from build123d import *

# Parameters (mm, degrees)
F_10_0MM_DOWEL_HOLE1_D      = 15
F_10_0MM_DOWEL_HOLE1_DEPTH  = 12
CIRPATTERN1_COUNT           = 6
F_10_0MM_DOWEL_HOLE2_D      = 15
F_10_0MM_DOWEL_HOLE2_DEPTH  = 12
CIRPATTERN2_COUNT           = 6
BOSS_EXTRUDE1_REACH         = 220.918
BOSS_EXTRUDE1_END_RADIUS    = 75
SKETCH12_R                  = 45
F_10_0MM_DOWEL_HOLE3_REACH  = 287.526
F_10_0MM_DOWEL_HOLE3_BORE_R = 30
F_12_0MM_DOWEL_HOLE1_D      = 12
F_12_0MM_DOWEL_HOLE1_DEPTH  = 12
CIRPATTERN3_COUNT           = 6


with BuildPart() as part:
    # Sketch1 → Revolve1 (revolve)
    with BuildSketch(Plane.XY, mode=Mode.PRIVATE) as revolve1_sk:
        Polygon((-100, -52.5), (-100, -95), (-88, -95), (-88, -62.5), (-50, -62.5), (-50, -75), (50, -75), (50, -65), (74, -65), (74, -50), (88, -50), (88, -95), (100, -95), (100, -36), (54, -36), (54, -43.5), (37, -43.5), (37, -52.5), (-35, -52.5), (-35, -47.5), (-95, -47.5), (-95, -52.5), align=None)
    revolve(revolve1_sk.sketch.rotate(Axis((0, 0, 0), (1, 0, 0)), 270), axis=Axis((0, 0, 0), (1, 0, 0)))

    # Ø10.0mm Dowel Hole1
    with Locations(Plane(origin=(100, 0, 0), x_dir=(0, 0, -1), z_dir=(1, 0, 0))):
        with Locations((0, 75)):
            f_10_0mm_dowel_hole1 = Hole(F_10_0MM_DOWEL_HOLE1_D / 2, depth=F_10_0MM_DOWEL_HOLE1_DEPTH)

    # CirPattern1: Ø10.0mm Dowel Hole1 ×6 about axis
    cirpattern1_axis = Axis((0, 0, 0), (1, 0, 0))
    for i in range(1, CIRPATTERN1_COUNT):
        add(f_10_0mm_dowel_hole1.rotate(cirpattern1_axis, i * 360 / CIRPATTERN1_COUNT), mode=Mode.SUBTRACT)

    # Ø10.0mm Dowel Hole2
    with Locations(Plane.ZY.offset(100)):
        with Locations((75, 0)):
            f_10_0mm_dowel_hole2 = Hole(F_10_0MM_DOWEL_HOLE2_D / 2, depth=F_10_0MM_DOWEL_HOLE2_DEPTH)

    # CirPattern2: Ø10.0mm Dowel Hole2 ×6 about axis
    cirpattern2_axis = Axis((0, 0, 0), (1, 0, 0))
    for i in range(1, CIRPATTERN2_COUNT):
        add(f_10_0mm_dowel_hole2.rotate(cirpattern2_axis, i * 360 / CIRPATTERN2_COUNT), mode=Mode.SUBTRACT)



with BuildPart() as body_2:
    # Sketch7 → Revolve3 (revolve)
    with BuildSketch(Plane.XY, mode=Mode.PRIVATE) as revolve3_sk:
        Polygon((0, 155), (80, 155), (80, 143), (40, 143), (40, 91), (45, 91), (45, 75), (0, 75), align=None)
    revolve(revolve3_sk.sketch.rotate(Axis((0, 0, 0), (0, 1, 0)), 90), axis=Axis((0, 0, 0), (0, 1, 0)))


with BuildPart() as part_1:
    add(part.part)

    add(body_2.part)  # Boss-Extrude1 merges body 2
    # Boss-Extrude1: up to this cylinder (the profile starts outside it)
    boss_extrude1_end = Plane(origin=(0, 0, 0), z_dir=(-1, 0, 0)) * Cylinder(BOSS_EXTRUDE1_END_RADIUS, 592.836, mode=Mode.PRIVATE)
    # Sketch12 → Boss-Extrude1 (add, up to the surface)
    with BuildSketch(Plane.XZ.offset(-75), mode=Mode.PRIVATE) as boss_extrude1_sk1:
        with Locations(Location((0, 0, 0), (0, 0, 90))):
            Circle(SKETCH12_R)
    boss_extrude1_tool1 = extrude(boss_extrude1_sk1.sketch, amount=BOSS_EXTRUDE1_REACH, mode=Mode.PRIVATE) - boss_extrude1_end
    add(boss_extrude1_tool1.solids().sort_by_distance((0, 75, 0))[0])
    add(boss_extrude1_tool1.solids().sort_by_distance((0, 75, 0))[1])

    # Ø10.0mm Dowel Hole3 bore → Ø10.0mm Dowel Hole3 (cut, up to next)
    with BuildSketch(Plane(origin=(0, 155, 0), x_dir=(1, 0, 0), z_dir=(0, 1, 0)), mode=Mode.PRIVATE) as f_10_0mm_dowel_hole3_sk1:
        Circle(F_10_0MM_DOWEL_HOLE3_BORE_R)
    f_10_0mm_dowel_hole3_tool1 = extrude(f_10_0mm_dowel_hole3_sk1.sketch, amount=-F_10_0MM_DOWEL_HOLE3_REACH, mode=Mode.PRIVATE) & part_1.part
    add(f_10_0mm_dowel_hole3_tool1.solids().sort_by_distance((0, 155, 0))[0], mode=Mode.SUBTRACT)

    # Ø12.0mm Dowel Hole1
    with Locations(Plane(origin=(-57.25292317, 155, 0), x_dir=(0, 0, 1), z_dir=(0, 1, 0))):
        with Locations((0, 0)):
            f_12_0mm_dowel_hole1 = Hole(F_12_0MM_DOWEL_HOLE1_D / 2, depth=F_12_0MM_DOWEL_HOLE1_DEPTH)

    # CirPattern3: Ø12.0mm Dowel Hole1 ×6 about axis
    cirpattern3_axis = Axis((0, 0, 0), (0, 1, 0))
    for i in range(1, CIRPATTERN3_COUNT):
        add(f_12_0mm_dowel_hole1.rotate(cirpattern3_axis, i * 360 / CIRPATTERN3_COUNT), mode=Mode.SUBTRACT)


solid = part_1.part
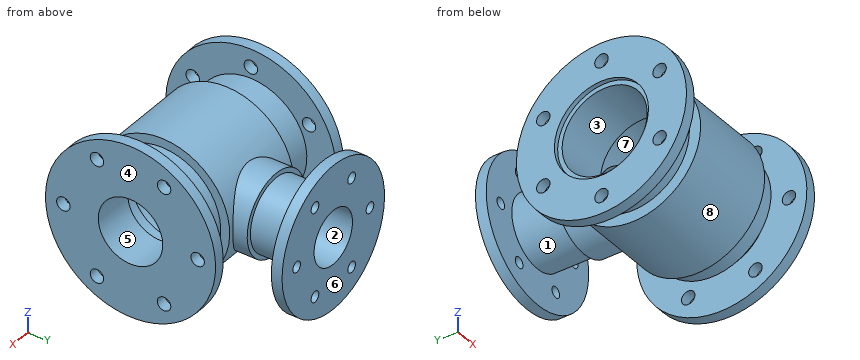
Source: CAD feature listing. Evaluate the final solid. Frame: model axes, mm. Face numbers are marked on the shaded views. A direction names the side the tool comes from. Round coordinates to 2 decimals unless told otherwise and drop trailing zeros. Write each loop counter-clockwise with the first axis right and the second up, starting at its lowest first coordinate (ties: lowest second). Pieces come first, ordered by that corner, then holes. Notation, with made-up numbers: (-21, 39) - (21, 39) arc R9 cw to (21, 49) - close; hole circle Ø9 at (56, 49). An arc over 180 degrees is marked (long way). Use CSV: the item, a comma, the result in double quotes. Start each with the question number.
(1) Material intervals for probe 1 along Y at (x, z) = (-71, 0); probe 2 along Y at (x, z) = (-44.5, 0.5); probe 3 along X at (y, z) = (-20.5, -72), sorted ascending. Write a range as [from, to].
(2) Cut plane D-D, the plane y = 117. Return loops of the section in (x, z), and give its area (3 significant figures).
(3) Set-up query: the marked faces 1, 2, 3, 4 and 5. Return all of +Z, -Z, +X, -X, +Y, -Y with unobstructed straight access to the full face (end or side cutting, diameter ignored); none if empty.
(4) Cut plane A-A, the plane y = 0. Give the number of separate pieces and of enclosed holes in the cut face, and give its area (3 significant figures).
(5) Mould query, pull axis Z, two halves, no side actions, for the marked faces 6, 7 and 8. Classes: pulls with the +Z half, pulls with the -Z half, needs draft (parallel to the pull), parting line crosses it, or undercut.
(6) Cut plane B-B, the plane x = 18.5. Return loops of the section in (y, z).
(7) First-contact query: pin 1 Ø4 at (y, z) = (-47, 10.5) entering from -X; pin 2 Ø5 at (x, z) = (-76.5, 19) entering from -Y; pin 3 Ø13.5 at (y, z) = (-64.95, -37.5) entering from -X. Flat tips, straight axial feed; report the tip coordinate or a pass-through.
Geometry says:
1,probe 1,"[-62.5, -47.5], [47.5, 62.5], [143, 155]"
1,probe 2,"[-75, -47.5], [47.5, 91], [143, 155]"
1,probe 3,"[-100, -88], [-50, 50], [88, 100]"
2,outline,"circle Ø80 at (0, 0); hole circle Ø60 at (0, 0)"
2,area,"2,200 mm²"
3,face 1,"none"
3,face 2,"+Y"
3,face 3,"-X"
3,face 4,"+Z, -Z, +X, +Y, -Y"
3,face 5,"+X, -X"
4,separate pieces,"4"
4,enclosed holes,"0"
4,area,"9,890 mm²"
5,face 6,"needs draft"
5,face 7,"undercut"
5,face 8,"parting line crosses it"
6,outline,"(46.89, -23.62) arc R52.5 cw (long way) to (46.89, 23.62) - (155, 23.62) - (155, 77.83) - (143, 77.83) - (143, 35.46) - (91, 35.46) - (91, 41.02) - (62.79, 41.02) arc R75 ccw (long way) to (62.79, -41.02) - (91, -41.02) - (91, -35.46) - (143, -35.46) - (143, -77.83) - (155, -77.83) - (155, -23.62) - close"
7,pin 1,"x = -95"
7,pin 2,"y = -60.28"
7,pin 3,"x = -50"
